Design review of the part shown in the three views and the two pictorial views. Dimensions are in mm from the part's minimum x, y and z. A direction names the side the tool comes from. Coordinates: 2 decimals unless noted, no trailing zeros. Loops run counter-clockwise (first coordinate to the right, second up) from the corner with the lowest first, then second, coordinate; pieces in that order, holes last.
Q1. Draft analysis for pull direction Y (two halves, no side actions). For the marked faces 1, 2 and 3, state which applies: released by +Y, released by -Y, zero draft, split by the parting line, or undercut.
Q2. Add section D-D on z = 20. Give the boundary of the cut face in (x, y), and give its area (3 significant figures).
Q3. For P1, Ø12, axis at y = 58, z = 9.5, coming from the -X side; P2, Ø19, axis at y = 48, z = 38.5, coming from the -X side; P3, Ø3, axis at x = 65, y = 42, coming from the +Z side; P4, Ø2, axis at x = 103, y = 43, coming from the +Z side, all flat-tipped, find the tip position at first contact; note any pin that passes through.
Q4. Wall thickness on probe 1 along X at (y, z) = (45, 18); probe 2 along Y at (x, z) = (46.5, 47); probe 3 along Z at (x, y) = (24.5, 67.5): over which ranges is each line inside the solid? List them lowest first.
Q5. Add section B-B on y = 8.5. Give the boundary of the cut face in (x, z), and give its area (3 significant figures).
Q6. Add section C-C on x = 28. Give the boundary of the cut face in (y, z).
Q7. Machinability: for the marked faces 4, 5 and 6, which of the approach directions +Z, -Z, +X, -X, +Y, -Y give a long, thin tool a straight path to every point of the face, cutting with its end or side? Answer none if there is none.
Q8. Add section A-A on x = 134. Give the boundary of the cut face in (y, z).
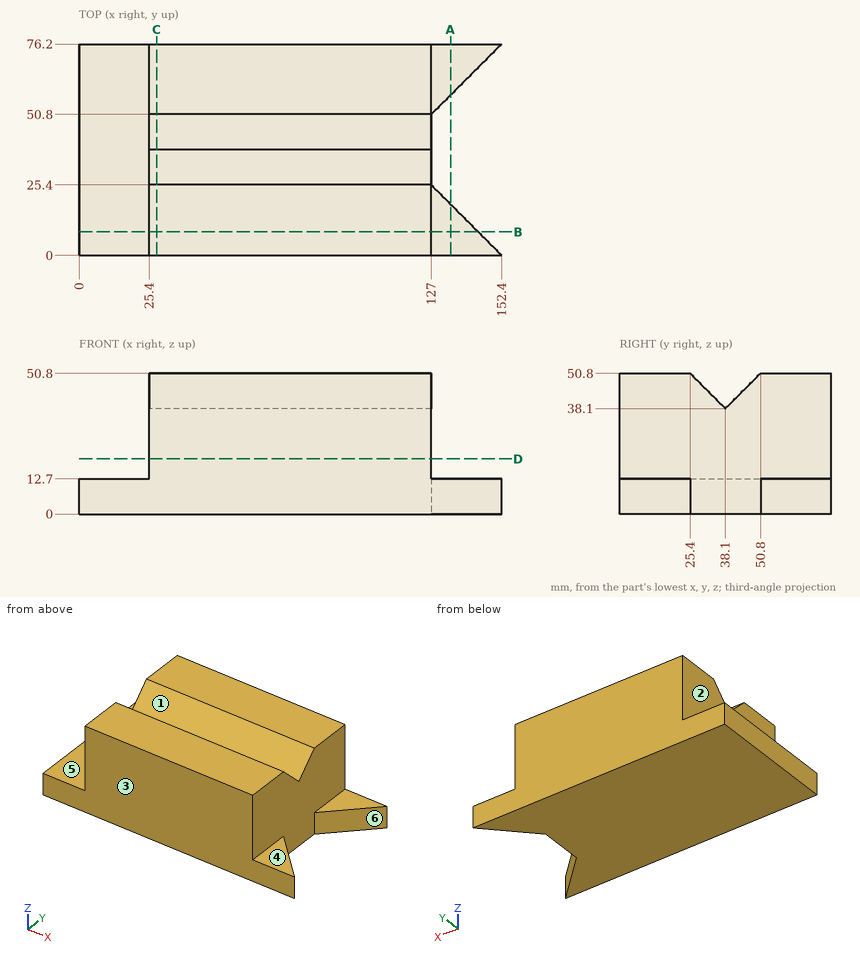
Entries:
1. face 1: undercut
1. face 2: zero draft
1. face 3: released by -Y
2. outline: (25.4, 0) - (127, 0) - (127, 76.2) - (25.4, 76.2) - close
2. area: 7,740 mm2
3. P1: stops at x = 0
3. P2: stops at x = 25.4
3. P3: stops at z = 43.5
3. P4: stops at z = 44
4. probe 1: x = 25.4 to 127
4. probe 2: y = 0 to 29.2, 47 to 76.2
4. probe 3: z = 0 to 12.7
5. outline: (0, 0) - (143.9, 0) - (143.9, 12.7) - (127, 12.7) - (127, 50.8) - (25.4, 50.8) - (25.4, 12.7) - (0, 12.7) - close
5. area: 5,700 mm2
6. outline: (0, 0) - (76.2, 0) - (76.2, 50.8) - (50.8, 50.8) - (38.1, 38.1) - (25.4, 50.8) - (0, 50.8) - close
7. face 4: +Z, +X, +Y, -Y
7. face 5: +Z, -X, +Y, -Y
7. face 6: +Z, -Z, +X
8. outline: (0, 0) - (18.4, 0) - (18.4, 12.7) - (0, 12.7) - close; (57.8, 0) - (76.2, 0) - (76.2, 12.7) - (57.8, 12.7) - close
